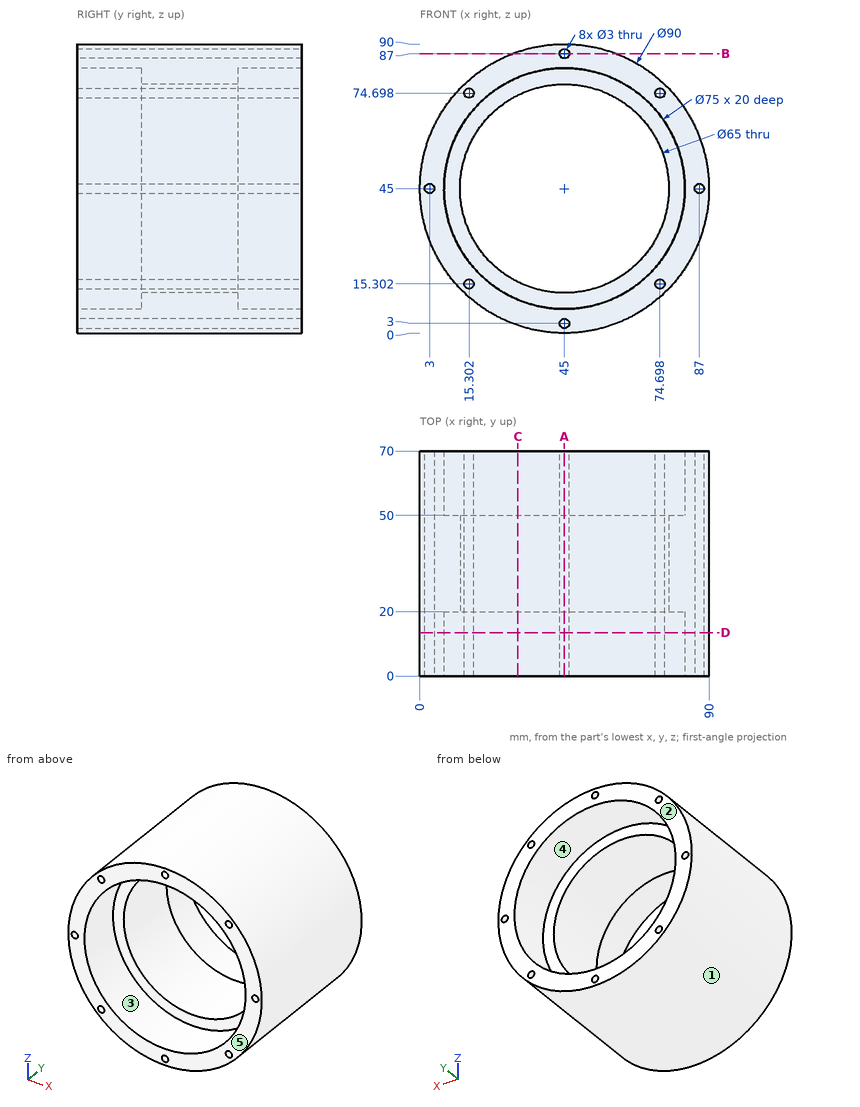
Verification items for this drawing (mm, ordinates from the low corner). A direction names the side the tool comes from. Round coordinates to 2 decimals unless told otherwise and drop trailing zeros. Loops run counter-clockwise (first coordinate to the right, second up) from the corner with the lowest first, then second, coordinate; pieces in that order, holes last. Notation, with made-up numbers: (-27, 45) -> (-9, 45) arc R15 cw to (-9, 60) -> close; hole circle Ø6 at (-13, 53). An arc over 180 degrees is marked (long way). Answer in a Markdown table with one row per item.
Q1. Set-up check for the marked faces 4 and 5: record each of +Z, -Z, +X, -X, +Y, -Y from which the full face is reachable in a straight line by a thin tool's end or side.
Data:
| item | result |
|---|---|
| face 4 | +Y |
| face 5 | +Z, -Z, +X, -X, -Y |
Q2. Sectioned sample at C-C on x = 30.5. Enter the section's corners in (y, z).
Data:
| item | result |
|---|---|
| outline | (0, 2.4) -> (70, 2.4) -> (70, 10.42) -> (50, 10.42) -> (50, 15.91) -> (20, 15.91) -> (20, 10.42) -> (0, 10.42) -> close; (0, 79.58) -> (20, 79.58) -> (20, 74.09) -> (50, 74.09) -> (50, 79.58) -> (70, 79.58) -> (70, 87.6) -> (0, 87.6) -> close |
Q3. Go/stop test with flat-tipped pins: P1, Ø2.5, axis at x = 15.3, z = 74.7, coming from the -Y side; P2, Ø4, axis at x = 32, y = 30, coming from the +Z side (1 decimal); P3, Ø3, axis at x = 21, z = 71.5, coming from the -Y side; P4, Ø3, axis at x = 10.5, y = 13.5, coming from the +Z side (1 decimal). Record where each tip stops, or that it passes through.
Data:
| item | result |
|---|---|
| P1 | passes through |
| P2 | stops at z = 88.6 |
| P3 | stops at y = 20 |
| P4 | stops at z = 75.6 |
Q4. Release check for a two-part mould opening along Z. For the marked faces 1, 2 and 3 record: released by +Z, released by -Z, zero draft, split by the parting line, or undercut.
Data:
| item | result |
|---|---|
| face 1 | split by the parting line |
| face 2 | zero draft |
| face 3 | undercut |
Q5. Sectioned sample at A-A on x = 45. Enter the section's corners in (y, z).
Data:
| item | result |
|---|---|
| outline | (0, 0) -> (70, 0) -> (70, 1.5) -> (0, 1.5) -> close; (0, 4.5) -> (70, 4.5) -> (70, 7.5) -> (50, 7.5) -> (50, 12.5) -> (20, 12.5) -> (20, 7.5) -> (0, 7.5) -> close; (0, 82.5) -> (20, 82.5) -> (20, 77.5) -> (50, 77.5) -> (50, 82.5) -> (70, 82.5) -> (70, 85.5) -> (0, 85.5) -> close; (0, 88.5) -> (70, 88.5) -> (70, 90) -> (0, 90) -> close |
Q6. Sectioned sample at B-B on z = 87. Enter the section's corners in (x, y) (1 decimal), then the cut area to 3 significant figures.
Data:
| item | result |
|---|---|
| outline | (28.8, 0) -> (43.5, 0) -> (43.5, 70) -> (28.8, 70) -> close; (46.5, 0) -> (61.2, 0) -> (61.2, 70) -> (46.5, 70) -> close |
| area | 2,050 mm^2 |
Q7. Thickness scan on L1, parallel to X at y = 52.5, z = 55.5; L2, parallel to X at y = 37.5, z = 70 (1 decimal); L3, parallel to Z at x = 47.5, y = 34. Record the ranges inside material, lowest first.
Data:
| item | result |
|---|---|
| L1 | x = 1.24 to 9, 81 to 88.76 |
| L2 | x = 7.6 to 24.2, 65.8 to 82.4 |
| L3 | z = 0.07 to 12.6, 77.4 to 89.93 |
Q8. Sectioned sample at D-D on y = 13.5. Give the number of separate pieces and of enclosed holes in the cut face, then the cut area to 3 significant figures.
Data:
| item | result |
|---|---|
| separate pieces | 1 |
| enclosed holes | 9 |
| area | 1,890 mm^2 |
